from build123d import *

# Parameters (mm, degrees)
SKETCH1_W           = 108.7
SKETCH1_H           = 300
BOSS_EXTRUDE1_DEPTH = 7.5
SKETCH2_W           = 65
SKETCH2_H           = 85
CUT_EXTRUDE1_DEPTH  = 7.5
CUT_EXTRUDE2_DEPTH  = 7.5
SKETCH5_W           = 30
SKETCH5_H           = 69
CUT_EXTRUDE3_DEPTH  = 7.5
SKETCH6_W           = 26
SKETCH6_H           = 80
CUT_EXTRUDE4_DEPTH  = 7.5
SKETCH9_W           = 17
SKETCH9_H           = 33
CUT_EXTRUDE5_DEPTH  = 7.5
SKETCH10_W          = 17
SKETCH10_H          = 10
CUT_EXTRUDE6_DEPTH  = 7.5
FILLET3_R           = 5
FILLET4_R           = 6


with BuildPart() as part:
    # Sketch1 → Boss-Extrude1 (new body)
    with BuildSketch(Plane.XY):
        Rectangle(SKETCH1_W, SKETCH1_H)
    extrude(amount=BOSS_EXTRUDE1_DEPTH)

    # Sketch2 → Cut-Extrude1 (cut)
    with BuildSketch(Plane.XY.offset(7.5)):
        with Locations((-21.85, 107.5)):
            Rectangle(SKETCH2_W, SKETCH2_H)
    extrude(amount=-CUT_EXTRUDE1_DEPTH, mode=Mode.SUBTRACT)

    # Sketch4 → Cut-Extrude2 (cut)
    with BuildSketch(Plane.XY.offset(7.5)):
        with BuildLine():
            Line((-54.35, 65), (-54.35, -34.475529761))
            ThreePointArc((-54.35, -34.475529761), (-25.449157059, 13.098498105), (-5.32998831, 65))
            Line((-5.32998831, 65), (-54.35, 65))
        make_face()
    extrude(amount=-CUT_EXTRUDE2_DEPTH, mode=Mode.SUBTRACT)

    # Sketch5 → Cut-Extrude3 (cut)
    with BuildSketch(Plane.XY.offset(7.5)):
        with Locations((32.5, 107.5)):
            Rectangle(SKETCH5_W, SKETCH5_H)
    extrude(amount=-CUT_EXTRUDE3_DEPTH, mode=Mode.SUBTRACT)

    # Sketch6 → Cut-Extrude4 (cut)
    with BuildSketch(Plane.XY.offset(7.5)):
        with Locations((10.65, 15.262235119)):
            Rectangle(SKETCH6_W, SKETCH6_H)
    extrude(amount=-CUT_EXTRUDE4_DEPTH, mode=Mode.SUBTRACT)

    # Sketch9 → Cut-Extrude5 (cut)
    with BuildSketch(Plane.XY.offset(7.5)):
        with Locations((39, 15.262235119)):
            Rectangle(SKETCH9_W, SKETCH9_H)
    extrude(amount=-CUT_EXTRUDE5_DEPTH, mode=Mode.SUBTRACT)

    # Sketch10 → Cut-Extrude6 (cut)
    with BuildSketch(Plane.XY.offset(7.5)):
        with Locations((39, 43.512235119)):
            Rectangle(SKETCH10_W, SKETCH10_H)
        with Locations((39, -12.987764881)):
            Rectangle(SKETCH10_W, SKETCH10_H)
    extrude(amount=-CUT_EXTRUDE6_DEPTH, mode=Mode.SUBTRACT)

    # Fillet3
    fillet3_edges = [part.edges().sort_by_distance(p)[0] for p in [
        (10.65, 150, 3.75),
        (10.65, 65, 3.75),
        (-5.32998831, 65, 3.75),
        (-54.35, -34.475529761, 3.75),
        (47.5, 142, 3.75),
        (47.5, 73, 3.75),
        (17.5, 73, 3.75),
        (17.5, 142, 3.75),
        (23.65, 55.262235119, 3.75),
        (23.65, -24.737764881, 3.75),
        (-2.35, -24.737764881, 3.75),
        (-2.35, 55.262235119, 3.75),
        (54.35, -150, 3.75),
        (-54.35, -150, 3.75),
        (47.5, 31.762235119, 3.75),
        (47.5, -1.237764881, 3.75),
        (30.5, -1.237764881, 3.75),
        (30.5, 31.762235119, 3.75),
        (54.35, 150, 3.75),
    ]]
    fillet(fillet3_edges, radius=FILLET3_R)

    # Fillet4
    # the kernel refuses this fillet: 6 mm, written as the material it adds along each edge
    with BuildSketch(Plane(origin=(47.5, -17.987764881, 7.5), x_dir=(0, 1, 0), z_dir=(0, 0, -1)), Plane(origin=(47.5, -7.987764881, 7.5), x_dir=(-1, 0, 0), z_dir=(0, 0, -1)), Plane(origin=(30.5, -17.987764881, 7.5), x_dir=(1, 0, 0), z_dir=(0, 0, -1)), Plane(origin=(47.5, 38.512235119, 7.5), x_dir=(0, 1, 0), z_dir=(0, 0, -1)), Plane(origin=(30.5, 38.512235119, 7.5), x_dir=(1, 0, 0), z_dir=(0, 0, -1)), Plane(origin=(47.5, 48.512235119, 7.5), x_dir=(-1, 0, 0), z_dir=(0, 0, -1))) as fillet4_piece_1:
        with BuildLine():
            CenterArc((FILLET4_R, -FILLET4_R), FILLET4_R, 90, 90)
            Line((0, -FILLET4_R), (0, 0))
            Line((0, 0), (FILLET4_R, 0))
        make_face()
    extrude(amount=7.5)
    with BuildSketch(Plane(origin=(30.5, -7.987764881, 7.5), x_dir=(1, 0, 0), z_dir=(0, 0, -1)), Plane(origin=(30.5, 48.512235119, 7.5), x_dir=(1, 0, 0), z_dir=(0, 0, -1))) as fillet4_piece_2:
        with BuildLine():
            CenterArc((FILLET4_R, FILLET4_R), FILLET4_R, 180, 90)
            Line((0, FILLET4_R), (0, 0))
            Line((0, 0), (FILLET4_R, 0))
        make_face()
    extrude(amount=7.5)


solid = part.part
The listing builds one solid part. Answer for the finished solid, in the listing's coordinates (mm). A direction names the side the tool comes from. Coordinates: 2 decimals unless noted, no trailing zeros. Write each loop counter-clockwise with the first axis right and the second up, starting at its lowest first coordinate (ties: lowest second). Pieces come first, ordered by that corner, then holes. Notation, with made-up numbers: (38, 39.25) - (78, 39.25) arc R34 ccw to (78, 70.25) - close; hole circle Ø9 at (-8, -6). An arc over 180 degrees is marked (long way). Return JSON: item names as keys, results as strings.
1. The part is cut by section C-C on x = -21. Determine the outline of the cut face in (y, z).
Final values:
{"outline": "(-150, 0) - (22.51, 0) - (22.51, 7.5) - (-150, 7.5) - close"}
2. For a pull along Y with two mould halves and no side action, classify faces 3 (the face through (45.42, -16.53, 3.8)), 4 (the face through (13, -31, 7.5)), 5 (the face through (52.92, 148.5, 3.8)) as +Y half, -Y half, draft (parallel to the pull), parting line (faces both ways), or undercut.
Final values:
{"face 3": "undercut", "face 4": "draft", "face 5": "+Y half"}
3. Consider line 1 along Y through (x, z) = (35, 1); line 2 along X through (y, z) = (137.5, 2.5); line 3 along Y through (x, z) = (19.5, 5.25). Determine where each line is inside the solid, lowest interval first.
Final values:
{"line 1": "-150 to -17.8, -8.18 to -1.21, 31.74 to 38.7, 48.32 to 73, 142 to 150", "line 2": "10.65 to 17.53, 47.47 to 54.35", "line 3": "-150 to -24.66, 55.19 to 74, 141 to 150"}
4. The part is cut by section B-B on z = 4.25. Count the separate pieces of the cut face and the enclosed holes in it, then the cut area to 3 significant figures.
Final values:
{"separate pieces": "1", "enclosed holes": "5", "area": "19,300 mm^2"}
5. The part is cut by section D-D on y = 58. Determine the outline of the cut face in (x, z), then the cut area to 3 significant figures.
Final values:
{"outline": "(-7.44, 0) - (54.35, 0) - (54.35, 7.5) - (-7.44, 7.5) - close", "area": "463 mm^2"}
6. The part is cut by section A-A on y = 105.5. Determine the outline of the cut face in (x, z).
Final values:
{"outline": "(10.65, 0) - (17.5, 0) - (17.5, 7.5) - (10.65, 7.5) - close; (47.5, 0) - (54.35, 0) - (54.35, 7.5) - (47.5, 7.5) - close"}
7. Which of the six approach directions +Z, -Z, +X, -X, +Y, -Y give full straight-line access (tool end or side, diameter ignored) to faces 1 (the face through (-1, -150, 4)), 2 (the face through (32.672, 39.892, 3.802))?
Final values:
{"face 1": "+Z, -Z, +X, -X, -Y", "face 2": "+Z, -Z"}
8. Each of these flat-tipped pins is pushed along its axis until it touches: pin 1 Ø4 at (y, z) = (111.5, 3.5) entering from -X; pin 2 Ø2 at (y, z) = (1.5, 3) entering from -X; pin 3 Ø2 at (y, z) = (14.5, 2.5) entering from -X. Where does it stop, or does it pass through?
Final values:
{"pin 1": "x = 10.65", "pin 2": "x = -32.01", "pin 3": "x = -25.25"}
